Can you work these out from the model? Positions are in its coordinate system, mm. A direction names the side the tool comes from. Round coordinates to 2 decimals unless told otherwise and drop trailing zeros. Loops run counter-clockwise (first coordinate to the right, second up) from the corner with the lowest first, then second, coordinate; pieces in that order, holes last. Notation, with made-up numbers: M 60,29.25 L 82,29.25 A6 cw 82,35.25 Z; hole C -31.5,-13.5 d8. An arc over 180 degrees is marked long. Answer as CSV lines item,"result".
from build123d import *

# Parameters (mm, degrees)
F0_R     = 3.15
F1_DEPTH = 6
F3_START = 22.4
F2_R     = 3
F3_DEPTH = 8.6
F5_START = -52.7
F5_DEPTH = 11
F6_R     = 3
F7_R     = 2.99999


# Not quite as in the source:
# - a fillet or chamfer is up to 0.001 mm smaller than in the source, because OpenCascade refuses the exact size


with BuildPart() as f1:
    # F0 (on Top) → F1 (new body)
    with BuildSketch(Plane.XY):
        with BuildLine():
            Line((24.4793512434, 46.0903614521), (24.4793512434, 48.1638564268))
            ThreePointArc((24.4793512434, 48.1638564268), (21.3598687714, 46.599431642), (18.9135639574, 44.1106189618))
            ThreePointArc((18.9135639574, 44.1106189618), (27.6293512434, 27.3403614521), (36.3451385294, 44.1106189618))
            ThreePointArc((36.3451385294, 44.1106189618), (33.8988337153, 46.599431642), (30.7793512434, 48.1638564268))
            Line((30.7793512434, 48.1638564268), (30.7793512434, 46.0903614521))
            Line((30.7793512434, 46.0903614521), (27.6293512434, 46.0903614521))
            Line((27.6293512434, 46.0903614521), (24.4793512434, 46.0903614521))
        make_face()
        with Locations((27.6293512434, 37.9903614521)):
            Circle(F0_R, mode=Mode.SUBTRACT)
        with BuildLine():
            ThreePointArc((18.9135639574, 44.1106189618), (21.3598687714, 46.599431642), (24.4793512434, 48.1638564268))
            Line((24.4793512434, 48.1638564268), (24.4793512434, 61.3403614521))
            Line((24.4793512434, 61.3403614521), (16.9793512434, 56.9903614521))
            Line((16.9793512434, 56.9903614521), (16.9793512434, 48.1108582074))
            ThreePointArc((16.9793512434, 48.1108582074), (18.6903086712, 46.4704086219), (18.9135639574, 44.1106189618))
        make_face()
        with BuildLine():
            ThreePointArc((30.7793512434, 48.1638564268), (33.8988337153, 46.599431642), (36.3451385294, 44.1106189618))
            ThreePointArc((36.3451385294, 44.1106189618), (36.5683938155, 46.4704086219), (38.2793512434, 48.1108582074))
            Line((38.2793512434, 48.1108582074), (38.2793512434, 56.9903614521))
            Line((38.2793512434, 56.9903614521), (30.7793512434, 61.3403614521))
            Line((30.7793512434, 61.3403614521), (30.7793512434, 48.1638564268))
        make_face()
    extrude(amount=F1_DEPTH)

    # F2 (on Right) → F3 (join)
    with BuildSketch(Plane.YZ.offset(F3_START)):
        with Locations((56.8403841853, 3.0001187697)):
            Circle(F2_R)
    extrude(amount=F3_DEPTH)

    # F4 (on Front) → F5 (cut)
    with BuildSketch(Plane.XZ.offset(F5_START)):
        Polygon((30.2794827968, -0.6592939026), (30.2794827968, 3.0006368179), (30.2794827968, 6.7412233911), (24.9780313224, 6.7412233911), (24.9780313224, -0.6592939026), align=None)
    extrude(amount=-F5_DEPTH, mode=Mode.SUBTRACT)

    # F6
    f6_edges = [f1.edges().sort_by_distance(p)[0] for p in [
        (27.629351, 46.090361, 6),
    ]]
    fillet(f6_edges, radius=F6_R)

    # F7 (radius 3 in the source; OpenCascade refuses exactly that, so slightly less here)
    f7_edges = [f1.edges().sort_by_distance(p)[0] for p in [
        (27.629351, 46.090361, 0),
    ]]
    fillet(f7_edges, radius=F7_R)


solid = f1.part
Item 1: If we section it at D-D on y = 40.5: Write out the boundary of the cut face in (x, z).
Output:
outline,"M 17.28,0 L 25.73,0 L 25.73,6 L 17.28,6 Z; M 29.53,0 L 37.98,0 L 37.98,6 L 29.53,6 Z"
Item 2: Will this pin go through, and if not, where does the flat tip stop? pin 1 (8 mm diameter, centred on x = 27.63, y = 37.99, fed in from -Z).
Output:
pin 1,"stops at z = 0"
Item 3: If we section it at B-B on z = 1: Write out the boundary of the cut face in (x, y), then the cut area to 3 significant figures.
Output:
outline,"M 16.98,48.11 A3.4 cw 18.91,44.11 A10.65 ccw long 36.35,44.11 A3.4 cw 38.28,48.11 L 38.28,56.99 L 30.78,61.34 L 30.78,59.08 L 30.28,59.08 L 30.28,54.6 L 30.78,54.6 L 30.78,45.33 L 24.48,45.33 L 24.48,54.6 L 24.98,54.6 L 24.98,59.08 L 24.48,59.08 L 24.48,61.34 L 16.98,56.99 Z; hole C 27.63,37.99 d6.3"
area,"495 mm2"
Item 4: On a 3-axis mill with a long thin cutter (end or side, diameter ignored), from which of +Z, -Z, +X, -X, +Y, -Y can I reach the whole of each face in a straight line? I mean faces 1 (the face through (30.279, 57, 3)), 2 (the face through (24.479, 52, 3)), 3 (the face through (38.279, 52, 3)), 4 (the face through (27.59, 45.19, 5.14)), 5 (the face through (27.59, 45.19, 0.86)). Say none if no direction works.
Output:
face 1,"+Z, -Z, +Y"
face 2,"none"
face 3,"+Z, -Z, +X, +Y, -Y"
face 4,"+Z"
face 5,"-Z"
Item 5: If we section it at A-A on y = 53: Write out the boundary of the cut face in (x, z), then the cut area to 3 significant figures.
Output:
outline,"M 16.98,0 L 24.48,0 L 24.48,6 L 16.98,6 Z; M 30.78,0 L 38.28,0 L 38.28,6 L 30.78,6 Z"
area,"90.0 mm2"
Item 6: If I drill on line 1 along X through (y, z) = (56.5, 3.25); line 2 along X through (y, z) = (50, 1.5); line 3 along Y through (x, z) = (24.75, 4.75), over which ranges is the centre line in solid material (lowest first)? Write a range as from..to.
Output:
line 1,"x = 16.98..24.98, 30.28..38.28"
line 2,"x = 16.98..24.48, 30.78..38.28"
line 3,"y = 27.74..36.71, 39.27..45.53, 54.4..59.28"
Item 7: We'd pull the mould along X, two halves only. Please class faces 6 (the face through (24.978, 57, 3)), 7 (the face through (20.782, 59.196, 2.958)), 8 (the face through (27.304, 27.345, 2.958)), 9 (the face through (24.7, 53.9, 2.4)): released by +X, released by -X, zero draft, split by the parting line, or undercut.
Output:
face 6,"undercut"
face 7,"released by -X"
face 8,"split by the parting line"
face 9,"undercut"
